from build123d import *

# Parameters (mm, degrees)
F3_DEPTH = 25
F4_T     = -3
F4_2_T   = -3
F5_W     = 5
F5_H     = 5
F6_DEPTH = 5


with BuildPart() as f3:
    # F1 (on Front) → F3 (new body)
    with BuildSketch(Plane.XZ):
        Polygon((-40, 80), (-40, 0), (-20, 0), (-20, 50), (-8, 32), (0, 32), (8, 32), (20, 50), (20, 0), (40, 0), (40, 80), (20, 80), (0, 50), (-20, 80), align=None)
    extrude(amount=F3_DEPTH)

    # F4
    f4_openings = [f3.faces().sort_by_distance(p)[0] for p in [
        (0, -25, 43.055762),
    ]]
    offset(amount=F4_T, openings=f4_openings, kind=Kind.INTERSECTION)



with BuildPart() as f3b:
    # F2 (on Front) → F3, piece 2 (new body)
    with BuildSketch(Plane.XZ):
        with BuildLine():
            Line((-40, 100), (-40, 85))
            Line((-40, 85), (60, 85))
            ThreePointArc((60, 85), (80, 65), (60, 45))
            Line((60, 45), (45, 45))
            Line((45, 45), (45, 30))
            Line((45, 30), (60, 30))
            ThreePointArc((60, 30), (95, 65), (60, 100))
            Line((60, 100), (-40, 100))
        make_face()
    extrude(amount=F3_DEPTH)

    # F4#2
    f4_2_openings = [f3b.faces().sort_by_distance(p)[0] for p in [
        (-38.479309, -25, 92.5),
    ]]
    offset(amount=F4_2_T, openings=f4_2_openings)


with BuildPart() as f3_1:
    add(f3.part)

    add(f3b.part)  # F6 merges F3b
    # F5 (on offset) → F6 (join)
    with BuildSketch(Plane.XY.offset(80)):
        with Locations((-30, -12.5)):
            Rectangle(F5_W, F5_H)
        with Locations((30, -12.5)):
            Rectangle(F5_W, F5_H)
    extrude(amount=F6_DEPTH)


solid = f3_1.part
The listing builds one solid part. Answer for the finished solid, in the listing's coordinates (mm). A direction names the side the tool comes from. Give positions to 0.01 mm unless a question says otherwise; leave off trailing zeros. Write each loop counter-clockwise with the first axis right and the second up, starting at its lowest first coordinate (ties: lowest second). Pieces come first, ordered by that corner, then holes. Notation, with made-up numbers: (39, 67) -> (63, 67) arc R34 ccw to (63, 98) -> close; hole circle Ø9 at (76.25, -2.75). An arc over 180 degrees is marked (long way). Use a Markdown table: item, result.
(1) Section B-B, the plane y = -20.5 is taken. Give the number of separate pieces and of enclosed holes in the cut face, then the cut area to 3 significant figures.
Return value:
| item | result |
|---|---|
| separate pieces | 2 |
| enclosed holes | 2 |
| area | 2,680 mm2 |
(2) Flat-ended cylindrical pins translate along their axes: P1, Ø13, axis at x = 3, y = -17.5, coming from the -Z side; P2, Ø2.5, axis at y = -14.5, z = 91.5, coming from the +X side; P3, Ø6, axis at y = -6, z = 70, coming from the +X side. Find the tip coordinate at first contact, or state that the pin passes through.
Return value:
| item | result |
|---|---|
| P1 | z = 32 |
| P2 | x = 84.24 |
| P3 | x = 94.94 |
(3) Find the intervals of material crossed by probe 1 along X at (y, z) = (-14, 12.5); probe 2 along Z at (x, y) = (36, -17.25); probe 3 along Z at (x, y) = (58.5, -15.75), in increasing order. Write a range as from..to.
Return value:
| item | result |
|---|---|
| probe 1 | -40..-37, -23..-20, 20..23, 37..40 |
| probe 2 | 0..3, 77..80, 85..88, 97..100 |
| probe 3 | 30..33, 42..45, 85..88, 97..100 |
(4) Section A-A, the plane z = 70 is taken. Determine the outline of the cut face in (x, y), then the cut area to 3 significant figures.
Return value:
| item | result |
|---|---|
| outline | (-40, -25) -> (-37, -25) -> (-37, -3) -> (-16.94, -3) -> (-16.94, -25) -> (-13.33, -25) -> (-13.33, 0) -> (-40, 0) -> close; (13.33, -25) -> (16.94, -25) -> (16.94, -3) -> (37, -3) -> (37, -25) -> (40, -25) -> (40, 0) -> (13.33, 0) -> close; (79.36, -25) -> (82.45, -25) -> (82.45, -3) -> (91.61, -3) -> (91.61, -25) -> (94.64, -25) -> (94.64, 0) -> (79.36, 0) -> close |
| area | 631 mm2 |
(5) Determine the mould class of faces 1 (the flat face through (-30, -15, 82)), 2 (the cylindrical face through (94.99, -12.32, 64.23)), 3 (the flat face through (10.95, -13.85, 61.02)) for opening direction X: released by +X, released by -X, zero draft, split by the parting line, or undercut.
Return value:
| item | result |
|---|---|
| face 1 | zero draft |
| face 2 | released by +X |
| face 3 | undercut |
(6) For faces 4 (the flat face through (0, -25, 46)), 5 (the flat face through (40, -12, 39)), 6 (the flat face through (27.5, -13, 82)), 7 (the flat face through (-10.65, -13.85, 60.57)), 8 (the flat face through (-30, -12, 0)), determine the directions among +Z, -Z, +X, -X, +Y, -Y from which every point of the face is accessible in a straight line to the end or side of a thin tool.
Return value:
| item | result |
|---|---|
| face 4 | +Z, -Z, +X, -X, -Y |
| face 5 | -Z, +Y, -Y |
| face 6 | +Y, -Y |
| face 7 | -Y |
| face 8 | -Z, +X, -X, +Y, -Y |
(7) Section C-C, the plane z = 11 is taken. Determine the outline of the cut face in (x, y).
Return value:
| item | result |
|---|---|
| outline | (-40, -25) -> (-37, -25) -> (-37, -3) -> (-23, -3) -> (-23, -25) -> (-20, -25) -> (-20, 0) -> (-40, 0) -> close; (20, -25) -> (23, -25) -> (23, -3) -> (37, -3) -> (37, -25) -> (40, -25) -> (40, 0) -> (20, 0) -> close |
